Read the model definition and answer for the solid it produces. Units are mm, in the model's axes. Face numbers are marked on the shaded views. A direction names the side the tool comes from. Round coordinates to 2 decimals unless told otherwise and drop trailing zeros. Order: outer loops, then holes, each group sorted by start corner. A loop starts at its lowest first (then second) coordinate and runs counter-clockwise, first axis right, second up. Notation, with made-up numbers: M -2.75,71 L 15.25,71 A14 ccw 15.25,77 Z; hole C -27.5,-10.75 d4. An arc over 180 degrees is marked long. Use one line per item in the form item = value. Start each with the question number.
from build123d import *

# Parameters (mm, degrees)
SKETCH1_R                = 1.5
BOSS_EXTRUDE1_DEPTH      = 9.22
BOSS_EXTRUDE2_DEPTH      = 12
SHELL1_START             = -10
SHELL1_OUTLINE_W         = 20.5
SHELL1_OUTLINE_H         = 16.44
SHELL1_DEPTH             = 27.5
SHELL1_START_2           = -29.5
SHELL1_2_DEPTH           = 14.5
SHELL1_START_3           = -16.5
SHELL1_3_DEPTH           = 1.5
SHELL1_START_4           = -8.22
SHELL1_4_DEPTH           = 16.44
SKETCH3_R                = 1.5
BOSS_EXTRUDE3_DEPTH      = 1
BOSS_EXTRUDE4_DEPTH      = 1.5
BOSS_EXTRUDE4_DEPTH_BACK = 1.5
SKETCH6_W                = 5
SKETCH6_H                = 5
SKETCH6_R                = 1.5
SKETCH7_R                = 2.75
CUT_EXTRUDE1_DEPTH       = 3
FILLET1_R                = 1
CUT_EXTRUDE2_DEPTH       = 20
CUT_EXTRUDE2_DEPTH_BACK  = 20
SKETCH8_R                = 0.956029162


with BuildPart() as part:
    # Sketch1 → Boss-Extrude1 (new, symmetric)
    with BuildSketch(Plane.XY):
        with BuildLine():
            Line((17.5, -11.25), (-17.5, -11.25))
            Line((-17.5, -11.25), (-17.5, 11.25))
            Line((-17.5, 11.25), (17.5, 11.25))
            ThreePointArc((17.5, 11.25), (18.914213562, 10.664213562), (19.5, 9.25))
            Line((19.5, 9.25), (19.5, -9.25))
            ThreePointArc((19.5, -9.25), (18.914213562, -10.664213562), (17.5, -11.25))
        make_face()
        with Locations((-12.5, 8.75)):
            Circle(SKETCH1_R, mode=Mode.SUBTRACT)
        with Locations((-12.5, -8.75)):
            Circle(SKETCH1_R, mode=Mode.SUBTRACT)
    extrude(amount=BOSS_EXTRUDE1_DEPTH, both=True)

    # Sketch2 → Boss-Extrude2 (add)
    with BuildSketch(Plane.ZY.offset(17.5)):
        with BuildLine():
            Line((9.22, -7.5), (9.22, 7.5))
            ThreePointArc((9.22, 7.5), (0, 11.25), (-9.22, 7.5))
            Line((-9.22, 7.5), (-9.22, -7.5))
            ThreePointArc((-9.22, -7.5), (0, -11.25), (9.22, -7.5))
        make_face()
    extrude(amount=BOSS_EXTRUDE2_DEPTH)

    # Shell1: read off the stored shape, not the designer's step
    # Shell1 outline → Shell1 (cut)
    with BuildSketch(Plane.YZ.offset(SHELL1_START)):
        Rectangle(SHELL1_OUTLINE_W, SHELL1_OUTLINE_H)
    extrude(amount=SHELL1_DEPTH, mode=Mode.SUBTRACT)

    # Shell1 2 outline → Shell1 2 (cut)
    with BuildSketch(Plane.YZ.offset(SHELL1_START_2)):
        with BuildLine():
            ThreePointArc((7.068411902, -8.22), (10.25, 0), (7.068411902, 8.22))
            Line((7.068411902, 8.22), (-7.068411902, 8.22))
            ThreePointArc((-7.068411902, 8.22), (-10.25, 0), (-7.068411902, -8.22))
            Line((-7.068411902, -8.22), (7.068411902, -8.22))
        make_face()
    extrude(amount=SHELL1_2_DEPTH, mode=Mode.SUBTRACT)

    # Shell1 3 outline → Shell1 3 (cut)
    with BuildSketch(Plane.YZ.offset(SHELL1_START_3)):
        with BuildLine():
            Line((10.25, 0), (10.25, 8.22))
            Line((10.25, 8.22), (7.068411902, 8.22))
            ThreePointArc((7.068411902, 8.22), (9.426855331, 4.407122157), (10.25, 0))
        make_face()
        with BuildLine():
            Line((10.25, -8.22), (10.25, 0))
            ThreePointArc((10.25, 0), (9.426855331, -4.407122157), (7.068411902, -8.22))
            Line((7.068411902, -8.22), (10.25, -8.22))
        make_face()
        with BuildLine():
            ThreePointArc((-10.25, 0), (-9.426855331, 4.407122157), (-7.068411902, 8.22))
            Line((-7.068411902, 8.22), (-10.25, 8.22))
            Line((-10.25, 8.22), (-10.25, 0))
        make_face()
        with BuildLine():
            Line((-10.25, -8.22), (-7.068411902, -8.22))
            ThreePointArc((-7.068411902, -8.22), (-9.426855331, -4.407122157), (-10.25, 0))
            Line((-10.25, 0), (-10.25, -8.22))
        make_face()
    extrude(amount=SHELL1_3_DEPTH, mode=Mode.SUBTRACT)

    # Shell1 4 outline → Shell1 4 (cut)
    with BuildSketch(Plane.XY.offset(SHELL1_START_4)):
        with BuildLine():
            ThreePointArc((-14.5, -10.25), (-14.871708245, -9.540569415), (-15, -8.75))
            Line((-15, -8.75), (-15, -10.25))
            Line((-15, -10.25), (-14.5, -10.25))
        make_face()
        with BuildLine():
            ThreePointArc((-10, 8.75), (-12.499999993, 6.25), (-15, 8.749999987))
            Line((-15, 8.749999987), (-15, -8.75))
            ThreePointArc((-15, -8.75), (-12.5, -6.25), (-10, -8.75))
            Line((-10, -8.75), (-10, 8.75))
        make_face()
        with BuildLine():
            Line((-14.5, 10.25), (-15, 10.25))
            Line((-15, 10.25), (-15, 8.749999987))
            ThreePointArc((-15, 8.749999987), (-14.871708247, 9.540569409), (-14.5, 10.25))
        make_face()
        with BuildLine():
            ThreePointArc((-10.5, 10.25), (-10.128291755, 9.540569415), (-10, 8.75))
            Line((-10, 8.75), (-10, 10.25))
            Line((-10, 10.25), (-10.5, 10.25))
        make_face()
        with BuildLine():
            Line((-10, -10.25), (-10, -8.75))
            ThreePointArc((-10, -8.75), (-10.128291755, -9.540569415), (-10.5, -10.25))
            Line((-10.5, -10.25), (-10, -10.25))
        make_face()
        with BuildLine():
            ThreePointArc((18.5, 9.25), (18.207106781, 9.957106781), (17.5, 10.25))
            Line((17.5, 10.25), (17.5, -10.25))
            ThreePointArc((17.5, -10.25), (18.207106781, -9.957106781), (18.5, -9.25))
            Line((18.5, -9.25), (18.5, 9.25))
        make_face()
    extrude(amount=SHELL1_4_DEPTH, mode=Mode.SUBTRACT)

    # Sketch3 → Boss-Extrude3 (add)
    with BuildSketch(Plane.ZY.offset(17.5)):
        with BuildLine():
            Line((-9.22, 7.5), (-9.22, -7.5))
            ThreePointArc((-9.22, -7.5), (0, -11.25), (9.22, -7.5))
            Line((9.22, -7.5), (9.22, 7.5))
            ThreePointArc((9.22, 7.5), (0, 11.25), (-9.22, 7.5))
        make_face()
        Circle(SKETCH3_R, mode=Mode.SUBTRACT)
    extrude(amount=BOSS_EXTRUDE3_DEPTH)

    # Sketch6 → Boss-Extrude4 (add, two sides: drawn at the far end of the back side and taken through both)
    with BuildSketch(Plane.XY.offset(-0.58).offset(-BOSS_EXTRUDE4_DEPTH_BACK)):
        with Locations((22, 0)):
            Rectangle(SKETCH6_W, SKETCH6_H)
        with Locations((22, 0)):
            Circle(SKETCH6_R, mode=Mode.SUBTRACT)
    extrude(amount=BOSS_EXTRUDE4_DEPTH + BOSS_EXTRUDE4_DEPTH_BACK)

    # Sketch7 → Cut-Extrude1 (cut)
    with BuildSketch(Plane.XY.offset(9.22)):
        with Locations((7.5, 0)):
            Circle(SKETCH7_R)
    extrude(amount=-CUT_EXTRUDE1_DEPTH, mode=Mode.SUBTRACT)

    # Fillet1
    fillet1_edges = [part.edges().sort_by_distance(p)[0] for p in [
        (19.5, 2.5, -0.58),
        (19.5, -2.5, -0.58),
    ]]
    fillet(fillet1_edges, radius=FILLET1_R)

    # Sketch8 → Cut-Extrude2 (cut, two sides: drawn at the far end of the back side and taken through both)
    with BuildSketch(Plane.XY.offset(-0.58).offset(-CUT_EXTRUDE2_DEPTH_BACK)):
        with Locations(Location((-16.061963922, 9.293970838, 0), (0, 0, 242.73008166))):
            Circle(SKETCH8_R)
        with Locations(Location((-16.061963922, -9.293970838, 0), (0, 0, 242.730056197))):
            Circle(SKETCH8_R)
    extrude(amount=CUT_EXTRUDE2_DEPTH + CUT_EXTRUDE2_DEPTH_BACK, mode=Mode.SUBTRACT)


solid = part.part
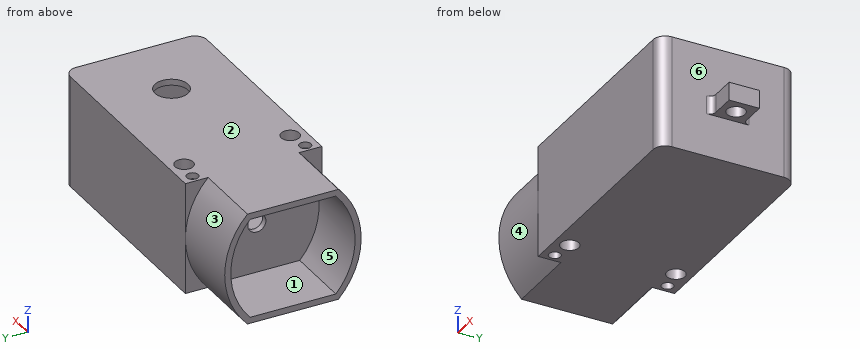
Item 1: For a pull along Z with two mould halves and no side action, classify the marked faces 4, 5 and 6 as pulls with the +Z half, pulls with the -Z half, needs draft (parallel to the pull), parting line crosses it, or undercut.
Item 2: Given P1, Ø5, axis at x = -23.5, z = -4.5, coming from the -Y side; P2, Ø2, axis at y = 1.5, z = -0.5, coming from the -X side; P3, Ø2, axis at y = 4, z = 6.5, coming from the +X side, each flat-ended and moving along its own axis, determine where each tip first touches the part or whether it passes through.
Item 3: A tool of negligible diameter and unlimited length cuts with its end or side. For the marked faces 1, 2 and 3, from which of +Z, -Z, +X, -X, +Y, -Y can it reach the whole face along a straight path? Write none if from no direction.
Item 4: Section B-B (x = 22) is taken. Write down the section's boundary in (y, z).
Item 5: Section D-D (y = 5.25) is taken. Write down the section's boundary in (x, z).
Item 6: Find the intervals of material crossed by L1, parallel to X at y = -2, z = -7.25; L2, parallel to Z at x = -20, y = -6.25; L3, parallel to Y at x = 13, z = 1.5, in increasing order. Write a range as [from, to].
Item 7: Section A-A (x = -12.5) is taken. Write down the section's boundary in (y, z).
Item 8: Section C-C (y = 0) is taken. Write down the section's boundary in (x, z), and give its area (3 significant figures).
The answers:
q1.face_4 = parting line crosses it
q1.face_5 = undercut
q1.face_6 = needs draft
q2.P1 = -11.1
q2.P2 = -18.5
q2.P3 = 19.5
q3.face_1 = -X
q3.face_2 = +Z, +X, -X, +Y, -Y
q3.face_3 = -X, +Y
q4.outline = M -2.5,-2.08 L -1.5,-2.08 L -1.5,0.92 L -2.5,0.92 Z; M 1.5,-2.08 L 2.5,-2.08 L 2.5,0.92 L 1.5,0.92 Z
q5.outline = M -29.5,-9.22 L 19.5,-9.22 L 19.5,9.22 L -29.5,9.22 L -29.5,8.22 L -18.5,8.22 L -18.5,-8.22 L -29.5,-8.22 Z; hole M -17.5,-8.22 L 18.5,-8.22 L 18.5,8.22 L -17.5,8.22 Z
q6.L1 = [-18.5, -17.5], [18.5, 19.5]
q6.L2 = [-9.22, -8.22], [8.22, 9.22]
q6.L3 = [-11.25, -10.25], [10.25, 11.25]
q7.outline = M -11.25,-9.22 L -10.25,-9.22 L -10.25,9.22 L -11.25,9.22 Z; M -7.25,-9.22 L 7.25,-9.22 L 7.25,9.22 L -7.25,9.22 Z; M 10.25,-9.22 L 11.25,-9.22 L 11.25,9.22 L 10.25,9.22 Z; hole M -6.25,-8.22 L 6.25,-8.22 L 6.25,8.22 L -6.25,8.22 Z
q8.outline = M -29.5,-9.22 L 19.5,-9.22 L 19.5,-2.08 L 20.5,-2.08 L 20.5,0.92 L 19.5,0.92 L 19.5,9.22 L 10.25,9.22 L 10.25,8.22 L 18.5,8.22 L 18.5,-8.22 L -17.5,-8.22 L -17.5,-1.5 L -18.5,-1.5 L -18.5,-8.22 L -29.5,-8.22 Z; M -29.5,8.22 L -18.5,8.22 L -18.5,1.5 L -17.5,1.5 L -17.5,8.22 L 4.75,8.22 L 4.75,9.22 L -29.5,9.22 Z; M 23.5,-2.08 L 24.5,-2.08 L 24.5,0.92 L 23.5,0.92 Z
q8.area = 128 mm²
